from build123d import *

# Parameters (mm, degrees)
SKETCH_1_R            = 27
EXTRUDE_360_DEPTH     = 9
SKETCH_2_R            = 16.175
CUT_EXTRUDE_445_DEPTH = 7
SKETCH_3_R            = 14
CUT_EXTRUDE_528_DEPTH = 39.820097888
SKETCH_4_R            = 1.65
CUT_EXTRUDE_687_DEPTH = 40.230090492
SKETCH_6_R            = 3.65
CUT_EXTRUDE_894_DEPTH = 3
SKETCH_7_R            = 3.5
EXTRUDE_1085_DEPTH    = 2
CHAMFER_1_SIZE        = 0.5


with BuildPart() as part:
    # Эскиз1 → Extrude 360 (new body)
    with BuildSketch(Plane.XY):
        Circle(SKETCH_1_R)
    extrude(amount=EXTRUDE_360_DEPTH)

    # Эскиз2 → Cut-Extrude 445 (cut)
    with BuildSketch(Plane.XY.offset(9)):
        Circle(SKETCH_2_R)
    extrude(amount=-CUT_EXTRUDE_445_DEPTH, mode=Mode.SUBTRACT)

    # Эскиз3 → Cut-Extrude 528 (cut, through all)
    with BuildSketch(Plane.XY.offset(2)):
        Circle(SKETCH_3_R)
    extrude(amount=-CUT_EXTRUDE_528_DEPTH, mode=Mode.SUBTRACT)

    # Эскиз4 → Cut-Extrude 687 (cut, through all)
    with BuildSketch(Plane.XY.offset(9)):
        with Locations((-18.186533479, 10.5)):
            Circle(SKETCH_4_R)
        with Locations((18.186533479, 10.5)):
            Circle(SKETCH_4_R)
        with Locations((0, -21)):
            Circle(SKETCH_4_R)
    extrude(amount=-CUT_EXTRUDE_687_DEPTH, mode=Mode.SUBTRACT)

    # Эскиз6 → Cut-Extrude 894 (cut)
    with BuildSketch(Plane(origin=(0, 0, 0), x_dir=(-1, 0, 0), z_dir=(0, 0, -1))):
        with Locations((0, 21)):
            Circle(SKETCH_6_R)
        with Locations((-18.186533479, -10.5)):
            Circle(SKETCH_6_R)
        with Locations((18.186533479, -10.5)):
            Circle(SKETCH_6_R)
    extrude(amount=-CUT_EXTRUDE_894_DEPTH, mode=Mode.SUBTRACT)

    # Эскиз7 → Extrude 1085 (add)
    with BuildSketch(Plane.XY.offset(9)):
        with Locations((0, 21)):
            Circle(SKETCH_7_R)
        with Locations((-18.186533479, -10.5)):
            Circle(SKETCH_7_R)
        with Locations((18.186533479, -10.5)):
            Circle(SKETCH_7_R)
    extrude(amount=EXTRUDE_1085_DEPTH)

    # Фаска1
    chamfer_1_edges = [part.edges().sort_by_distance(p)[0] for p in [
        (-3.5, 21, 11),
        (-21.686533479, -10.5, 11),
        (14.686533479, -10.5, 11),
    ]]
    chamfer(chamfer_1_edges, length=CHAMFER_1_SIZE)


solid = part.part
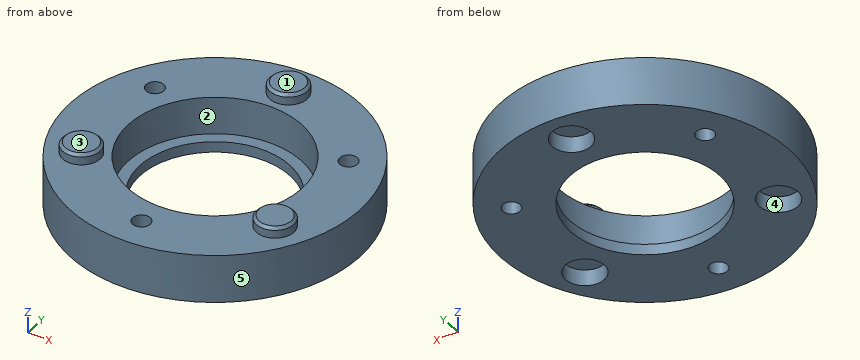
Input: part model. Units: mm. Frame: model coordinates. Face numbers are marked on the shaded views. A direction names the side the tool comes from. Give positions to 0.01 mm unless a question says otherwise; leave off trailing zeros. Loops run counter-clockwise (first coordinate to the right, second up) from the corner with the lowest first, then second, coordinate; pieces in that order, holes last. Notation, with made-up numbers: (51, 60.25) -> (84, 60.25) arc R19 cw to (84, 97.25) -> close; hole circle Ø1 at (0, 38). An arc over 180 degrees is marked (long way). Answer as a JSON object with one key per item and string values. Group by question number.
Item 1: Line query: probe 1 along Z at (x, y) = (-11.5, -18); probe 2 along Z at (x, y) = (-16, -0.5); probe 3 along Y at (x, z) = (-1.5, 8). Output: solid intervals per line, ascending.
Item 2: Pull-direction query (X, two-part tool) for the marked faces 3, 4 and 5; classes: released by +X, released by -X, zero draft, split by the parting line, or undercut.
Item 3: Cut plane D-D, the plane x = 13. Return the cut outline in (y, z), and give its area (3 significant figures).
Item 4: Cut plane C-C, the plane x = 0. Return the cut outline in (y, z) (3 decimals).
Item 5: Pin query (flat end, axial travel): P1, Ø3.5, axis at x = 19.5, y = -10, coming from the -Z side; P2, Ø10, axis at x = -19, y = 20.5, coming from the +Z side; P3, Ø22.5, axis at x = 0, y = 0, coming from the +Z side; P4, Ø6, axis at x = -7, z = 9.5, coming from the +Y side. Return the tip coordinate at first contact, or that it passes through.
Item 6: Reachability of the marked faces 1 and 2 from +Z, -Z, +X, -X, +Y, -Y: full face, straight path, thin tool, end or side. Return the list, or none.
Item 7: Cut plane A-A, the plane z = 1. Return the cut outline in (x, y), and give its area (3 significant figures).
Checks:
{
 "1": {"probe 1": "z = 0 to 9", "probe 2": "z = 0 to 2", "probe 3": "y = -26.96 to -21.69, -20.31 to -16.11, 16.11 to 26.96"},
 "2": {"face 3": "zero draft", "face 4": "undercut", "face 5": "split by the parting line"},
 "3": {"outline": "(-23.66, 0) -> (-5.2, 0) -> (-5.2, 2) -> (-9.62, 2) -> (-9.62, 9) -> (-23.66, 9) -> close; (5.2, 0) -> (23.66, 0) -> (23.66, 9) -> (9.62, 9) -> (9.62, 2) -> (5.2, 2) -> close", "area": "270 mm²"},
 "4": {"outline": "(-27, 0) -> (-22.65, 0) -> (-22.65, 9) -> (-27, 9) -> close; (-19.35, 0) -> (-14, 0) -> (-14, 2) -> (-16.175, 2) -> (-16.175, 9) -> (-19.35, 9) -> close; (14, 0) -> (17.35, 0) -> (17.35, 3) -> (24.65, 3) -> (24.65, 0) -> (27, 0) -> (27, 9) -> (24.5, 9) -> (24.5, 10.5) -> (24, 11) -> (18, 11) -> (17.5, 10.5) -> (17.5, 9) -> (16.175, 9) -> (16.175, 2) -> (14, 2) -> close"},
 "5": {"P1": "stops at z = 3", "P2": "stops at z = 9", "P3": "passes through", "P4": "stops at y = 26.7"},
 "6": {"face 1": "+Z, +X, -X, +Y, -Y", "face 2": "+Z"},
 "7": {"outline": "circle Ø54 at (0, 0); hole circle Ø7.3 at (-18.19, -10.5); hole circle Ø3.3 at (-18.19, 10.5); hole circle Ø28 at (0, 0); hole circle Ø7.3 at (0, 21); hole circle Ø3.3 at (0, -21); hole circle Ø7.3 at (18.19, -10.5); hole circle Ø3.3 at (18.19, 10.5)", "area": "1,520 mm²"}
}
